from build123d import *

# Parameters (mm, degrees)
SKETCH_W        = 50
SKETCH_H        = 12
PAD_DEPTH       = 20
POCKET_DEPTH    = 20
POCKET001_DEPTH = 10
SKETCH003_R     = 3.2
POCKET002_DEPTH = 5
SKETCH004_R     = 3.5
PAD001_DEPTH    = 20
SKETCH005_R     = 3.5
PAD002_DEPTH    = 20
FILLET_R        = 1
SKETCH006_R     = 1.15
POCKET003_DEPTH = 200
FILLET001_R     = 1


with BuildPart() as part:
    # Sketch → Pad (new body)
    with BuildSketch(Plane.XY):
        Rectangle(SKETCH_W, SKETCH_H)
    extrude(amount=PAD_DEPTH)

    # Sketch001 (on Face3 of Pad) → Pocket (cut)
    with BuildSketch(Plane.XZ.offset(6)):
        Polygon((-25, 30), (-25, 10), (-6, 20), (6, 20), (25, 10), (25, 30), align=None)
    extrude(amount=-POCKET_DEPTH, mode=Mode.SUBTRACT)

    # Sketch002 (on Face8 of Pocket) → Pocket001 (cut)
    with BuildSketch(Plane.XZ.offset(6)):
        Polygon((-15, 12), (-15, 3), (15, 3), (15, 12), (6, 17.5), (-6, 17.5), align=None)
    extrude(amount=-POCKET001_DEPTH, mode=Mode.SUBTRACT)

    # Sketch003 (on Face5 of Pocket001) → Pocket002 (cut)
    with BuildSketch(Plane.XY.offset(20)):
        Circle(SKETCH003_R)
    extrude(amount=-POCKET002_DEPTH, mode=Mode.SUBTRACT)

    # Sketch004 (on Face7 of Pocket002) → Pad001 (join)
    with BuildSketch(Plane(origin=(-25, 0, 0), x_dir=(0, -1, 0), z_dir=(-1, 0, 0))):
        with Locations((0, 6)):
            Circle(SKETCH004_R)
    extrude(amount=PAD001_DEPTH)

    # Sketch005 (on Face3 of Pad001) → Pad002 (join)
    with BuildSketch(Plane.YZ.offset(25)):
        with Locations((0, 6)):
            Circle(SKETCH005_R)
    extrude(amount=PAD002_DEPTH)

    # Fillet
    fillet_edges = [part.edges().sort_by_distance(p)[0] for p in [
        (25, -3.5, 6),
        (-25, 3.5, 6),
    ]]
    fillet(fillet_edges, radius=FILLET_R)

    # Sketch006 (on Face26 of Fillet) → Pocket003 (cut)
    with BuildSketch(Plane(origin=(-45, 0, 0), x_dir=(0, -1, 0), z_dir=(-1, 0, 0))):
        with Locations((0, 6)):
            Circle(SKETCH006_R)
    extrude(amount=-POCKET003_DEPTH, mode=Mode.SUBTRACT)

    # Fillet001
    fillet001_edges = [part.edges().sort_by_distance(p)[0] for p in [
        (-15.5, -6, 15),
        (-25, -6, 5),
        (-25, 6, 5),
        (-15.5, 6, 15),
        (15.5, -6, 15),
        (15.5, 6, 15),
        (25, -6, 5),
        (25, 6, 5),
    ]]
    fillet(fillet001_edges, radius=FILLET001_R)


solid = part.part
Verification items for the finished model (mm, model axes). A direction names the side the tool comes from. Coordinates: 2 decimals unless noted, no trailing zeros. Order: outer loops, then holes, each group sorted by start corner. A loop starts at its lowest first (then second) coordinate and runs counter-clockwise, first axis right, second up.
1. Scan lines: line 1 (Z direction, x = -33.5, y = 0); line 2 (X direction, y = -4.5, z = 4); line 3 (Y direction, x = 0, z = 18.35). Record each from-to range of solid material in increasing order.
Results found:
line 1: z = 2.5 to 4.85, 7.15 to 9.5
line 2: x = -25 to -15, 15 to 25
line 3: y = -6 to -3.2, 3.2 to 6
2. Set-up check for faces 1 (the face through (35.28, -0.759, 2.583)), 2 (the face through (-2.539, -1.947, 18.768)), 3 (the face through (0, 4, 10)): record each of +Z, -Z, +X, -X, +Y, -Y from which the full face is reachable in a straight line by a thin tool's end or side.
Results found:
face 1: +X
face 2: +Z
face 3: -Y
3. Release check for a two-part mould opening along Z. For faces 4 (the face through (0, -1, 3)), 5 (the face through (-15, -1, 8)), 6 (the face through (-35.28, 0.759, 2.583)), 7 (the face through (-45, 1, 7)) record: +Z half, -Z half, draft (parallel to the pull), parting line (faces both ways), or undercut.
Results found:
face 4: undercut
face 5: undercut
face 6: parting line
face 7: draft
4. Sectioned sample at B-B, the plane x = 0. Record the cut outline in (y, z).
Results found:
outline: (-6, 0) - (6, 0) - (6, 20) - (3.2, 20) - (3.2, 17.5) - (4, 17.5) - (4, 3) - (-6, 3) - close; (-6, 17.5) - (-3.2, 17.5) - (-3.2, 20) - (-6, 20) - close
5. Sectioned sample at D-D, the plane x = -32. Record the cut outline in (y, z).
Results found:
outline: circle Ø7 at (0, 6); hole circle Ø2.3 at (0, 6)
6. Sectioned sample at A-A, the plane z = 6. Give the number of separate pieces and of enclosed holes in the cut face, and give its area (3 significant figures).
Results found:
separate pieces: 3
enclosed holes: 0
area: 442 mm2
7. Go/stop test with flat-tipped pins: pin 1 Ø1.5 at (x, y) = (-17, -3) entering from +Z; pin 2 Ø3 at (x, z) = (13, 8) entering from -Y; pin 3 Ø2 at (x, y) = (8, -1) entering from +Z. Record where each tip stops, or that it passes through.
Results found:
pin 1: stops at z = 14.61
pin 2: stops at y = 4
pin 3: stops at z = 19.47
